Verification items for this drawing (mm, ordinates from the low corner). Coordinates: 2 decimals unless noted, no trailing zeros. Write each loop counter-clockwise with the first axis right and the second up, starting at its lowest first coordinate (ties: lowest second). Pieces come first, ordered by that corner, then holes. Notation, with made-up numbers: (80.5, 0) -> (117.5, 0) arc R6 ccw to (117.5, 10) -> close; hole circle Ø6 at (-5, 87.5). An arc over 180 degrees is marked (long way). One line per question, with ' | ' between items.
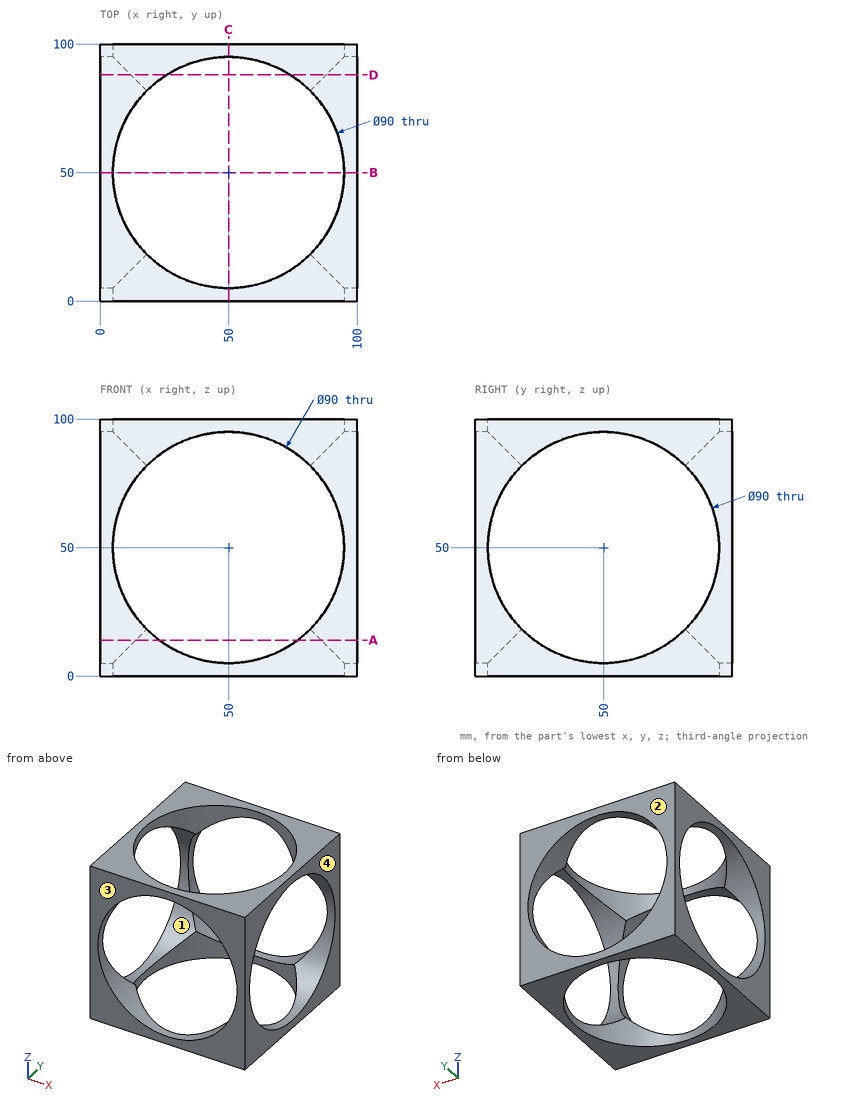
(1) Cross-section at A-A (z = 14). Record the cut outline in (x, y), plus the area to 3 significant figures.
Answers below:
outline: (0, 0) -> (23, 0) -> (23, 14) arc R45 cw to (14, 23) -> (0, 23) -> close; (0, 77) -> (14, 77) arc R45 cw to (23, 86) -> (23, 100) -> (0, 100) -> close; (77, 0) -> (100, 0) -> (100, 23) -> (86, 23) arc R45 cw to (77, 14) -> close; (77, 86) arc R45 cw to (86, 77) -> (100, 77) -> (100, 100) -> (77, 100) -> close | area: 1,940 mm²
(2) Draft check along Y on the marked faces 1, 2, 3 and 4. Enter one of: pulls with the +Y half, pulls with the -Y half, needs draft (parallel to the pull), parting line crosses it, or undercut.
Answers below:
face 1: undercut | face 2: pulls with the +Y half | face 3: pulls with the -Y half | face 4: needs draft
(3) Cross-section at B-B (y = 50). Record the cut outline in (x, z).
Answers below:
outline: (0, 0) -> (5, 0) -> (5, 5) -> (0, 5) -> close; (0, 95) -> (5, 95) -> (5, 100) -> (0, 100) -> close; (95, 0) -> (100, 0) -> (100, 5) -> (95, 5) -> close; (95, 95) -> (100, 95) -> (100, 100) -> (95, 100) -> close
(4) Cross-section at D-D (y = 88). Record the cut outline in (x, z), plus the area to 3 significant figures.
Answers below:
outline: (0, 0) -> (25.9, 0) -> (25.9, 12) arc R45 cw to (12, 25.9) -> (0, 25.9) -> close; (0, 74.1) -> (12, 74.1) arc R45 cw to (25.9, 88) -> (25.9, 100) -> (0, 100) -> close; (74.1, 0) -> (100, 0) -> (100, 25.9) -> (88, 25.9) arc R45 cw to (74.1, 12) -> close; (74.1, 88) arc R45 cw to (88, 74.1) -> (100, 74.1) -> (100, 100) -> (74.1, 100) -> close | area: 2,240 mm²
(5) Material ranges on line 1 (Y direction, x = 50, z = 4); line 2 (X direction, y = 31.5, z = 93), recorded low to high.
Answers below:
line 1: y = 0 to 5, 95 to 100 | line 2: x = 0 to 8.98, 91.02 to 100
